For this review, use the dimensioned drawing (mm, ordinates from the lowest corner) and the shaded views. A direction names the side the tool comes from. Round coordinates to 2 decimals unless told otherwise and drop trailing zeros. Loops run counter-clockwise (first coordinate to the right, second up) from the corner with the lowest first, then second, coordinate; pieces in that order, holes last. Notation, with made-up numbers: (6.5, -33) - (56.5, -33) arc R7 ccw to (56.5, -23) - close; hole circle Ø10 at (-2.5, 76.5). An arc over 180 degrees is marked (long way). Use one line per item in the form item = value. Start each with the question number.
(1) We need section A-A, the plane z = 23. Write out the cut boundary in (x, y) (3 decimals).
(2) For pin 1 (8 mm diameter, centred on x = 22, z = 23.5, fed in from -Y); pin 2 (1 mm diameter, centred on y = 25.5, z = 11.5, fed in from -X); pin 3 (4.5 mm diameter, centred on x = 26, y = 56, fed in from +Z); pin 4 (10 mm diameter, centred on y = 52.5, z = 5, fed in from +X), all flat-tipped, find the tip position at first contact; note any pin that passes through.
(3) We need section C-C, the plane y = 54.5. Write out the cut boundary in (x, z) (3 decimals).
(4) We need section B-B, the plane y = 6.35. Write out the cut boundary in (x, z) (3 decimals).
(5) Machinability: for the marked faces 4, 5, 6 and 7, which of the approach directions +Z, -Z, +X, -X, +Y, -Y give a long, thin tool a straight path to every point of the face, cutting with its end or side? Answer none if there is none.
(6) We need section D-D, the plane z = 31. Write out the cut boundary in (x, y) (3 decimals), then the cut area to 3 significant figures.
(7) The part is to be moulded in two halves that separate along X. For the marked faces 1, 2 and 3, say which applies: released by +X, released by -X, zero draft, split by the parting line, or undercut.
(8) Wall thickness on probe 1 along Y at (x, z) = (54, 19); probe 2 along X at (y, z) = (57, 27) (3 decimals); probe 3 along Z at (x, y) = (54.25, 6.35) (3 decimals): over which ranges is each line inside the solid? List them lowest first. Write a range as [from, to].
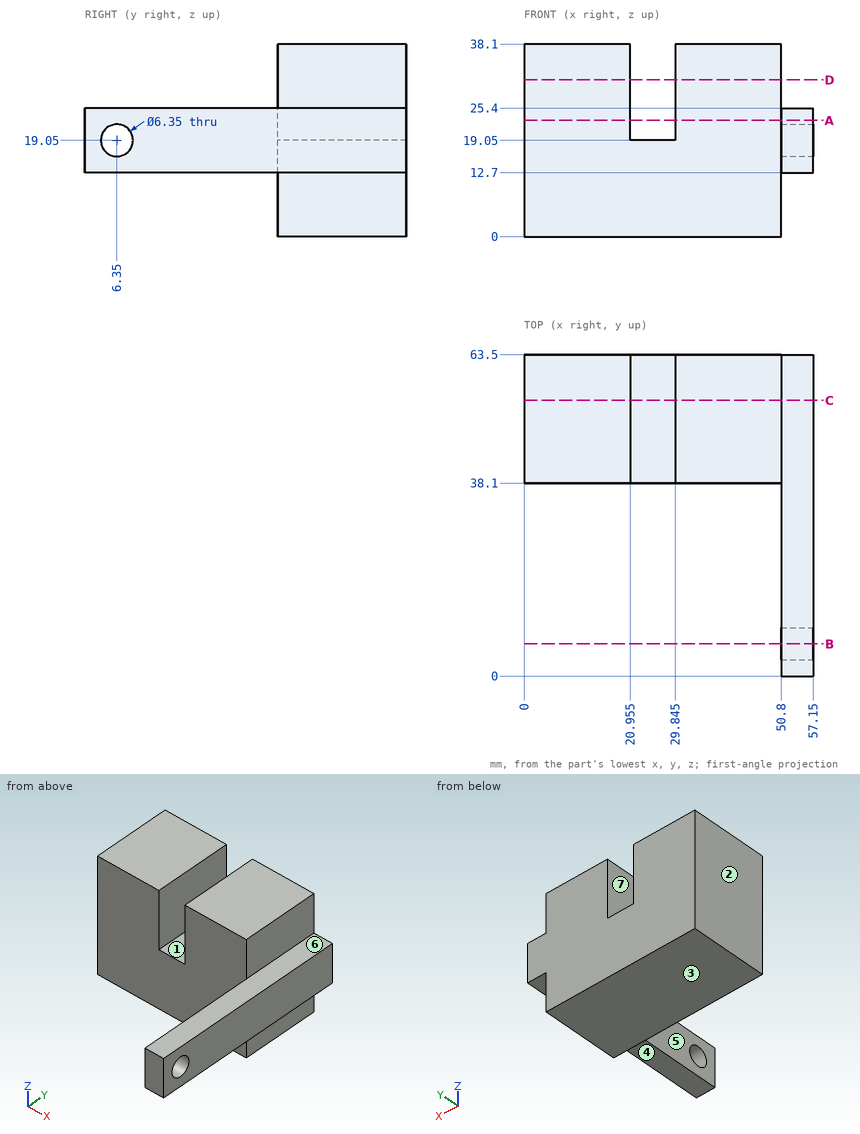
Data:
q1.outline = (0, 38.1) - (20.955, 38.1) - (20.955, 63.5) - (0, 63.5) - close; (29.845, 38.1) - (50.8, 38.1) - (50.8, 0) - (57.15, 0) - (57.15, 63.5) - (29.845, 63.5) - close
q2.pin_1 = 38.1
q2.pin_2 = through
q2.pin_3 = 19.05
q2.pin_4 = 50.8
q3.outline = (0, 0) - (50.8, 0) - (50.8, 12.7) - (57.15, 12.7) - (57.15, 25.4) - (50.8, 25.4) - (50.8, 38.1) - (29.845, 38.1) - (29.845, 19.05) - (20.955, 19.05) - (20.955, 38.1) - (0, 38.1) - close
q4.outline = (50.8, 12.7) - (57.15, 12.7) - (57.15, 15.875) - (50.8, 15.875) - close; (50.8, 22.225) - (57.15, 22.225) - (57.15, 25.4) - (50.8, 25.4) - close
q5.face_4 = -Z, +X, +Y, -Y
q5.face_5 = +Z, -Z, -X, -Y
q5.face_6 = +Z, +X, +Y, -Y
q5.face_7 = +Z, +Y, -Y
q6.outline = (0, 38.1) - (20.955, 38.1) - (20.955, 63.5) - (0, 63.5) - close; (29.845, 38.1) - (50.8, 38.1) - (50.8, 63.5) - (29.845, 63.5) - close
q6.area = 1,060 mm^2
q7.face_1 = undercut
q7.face_2 = released by -X
q7.face_3 = zero draft
q8.probe_1 = [0, 3.18], [9.52, 63.5]
q8.probe_2 = [0, 20.955], [29.845, 50.8]
q8.probe_3 = [12.7, 15.875], [22.225, 25.4]
